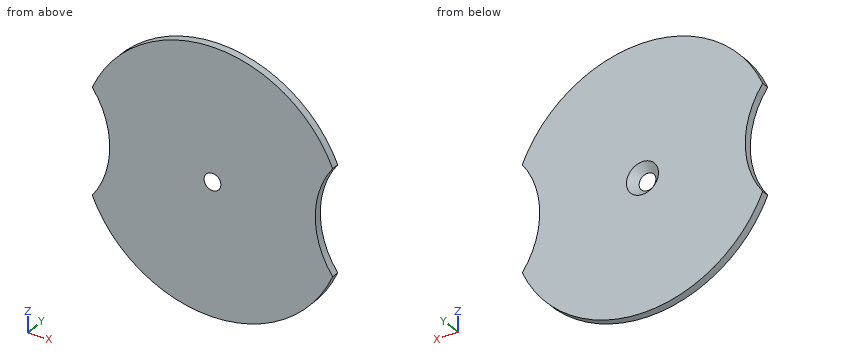
Autodesk Inventor part; units mm, degrees
ref_plane "YZ Plane" through (0, 0, 0) normal (1, 0, 0) x (0, 1, 0)
ref_plane "XZ Plane" through (0, 0, 0) normal (0, 1, 0) x (-1, 0, 0)
ref_plane "XY Plane" through (0, 0, 0) normal (0, 0, 1) x (1, 0, 0)
sketch "スケッチ1" plane through (0, 0, 0) normal (0, 1, 0) x (-1, 0, 0)
  line L0 (0, -24.08) -> (0, 24.08)
  line L1 (-51.0552, 0) -> (51.0552, 0)
  circle A0 centre (0, 0) radius 17.2
  circle A1 centre (0, 0) radius 1.1
  circle A2 centre (24.968, 0) radius 11.5
  circle A3 centre (-24.968, 0) radius 11.5
  line L2 (1.9153, -7.1479) -> (2.64, -9.8524)
  arc A4 (-1.9153, -7.1479) -> (1.9153, -7.1479) centre (0, 0) ccw
  line L3 (-1.9153, -7.1479) -> (-2.64, -9.8524)
  line L4 (0, -11) -> (0.5714, -10.184)
  line L5 (0, -11) -> (-0.5714, -10.184)
  arc A5 (-2.64, -9.8524) -> (-0.5714, -10.184) centre (0, 0) ccw
  arc A6 (0.5714, -10.184) -> (2.64, -9.8524) centre (0, 0) ccw
  point P0 (-15.76, 6.8893)
  point P1 (-15.76, -6.8893)
  point P2 (15.76, -6.8893)
  point P3 (15.76, 6.8893)
  dimension "d0" = 34.4
  dimension "d1" = 2.2
  dimension "d2" = 24.968
  dimension "d3" = 23
  dimension "d8" = 30
  dimension "d9" = 7.4
  dimension "d11" = 10.2
  dimension "d12" = 11
  dimension "d13" = 70
extrude "押し出し1" add sketch "スケッチ1" along normal blind 1 contours A0 A3 L1 A1 L0 A4 L3 A5 L5 | L0 L4 A6 L2 A4 A1 L1 A2 A0 | L5 A5 L3 A4 L0 | L0 A4 L2 A6 L4 | A3 A0 L0 A1 L1 | L1 A1 L0 A0 A2
chamfer "面取り1" distance 1 angle 45 1 edges at (1.1, 1, 0)
properties part number "GearCenterCover"
Here's how the part is built. I have some questions about the finished solid (model axes, mm). Coordinates: 2 decimals unless noted, no trailing zeros. Order: outer loops, then holes, each group sorted by start corner. A loop starts at its lowest first (then second) coordinate and runs counter-clockwise, first axis right, second up.
Item 1: If we section it at D-D, the plane x = -10.5: List the corners of the cut face in (y, z) for me.
Response values:
outline: (0, -13.62) - (1, -13.62) - (1, 13.62) - (0, 13.62) - close
Item 2: If we section it at B-B, the plane y = 0.7: List the corners of the cut face in (x, z) for me, then the cut area to 3 significant figures.
Response values:
outline: (-15.76, -6.89) arc R17.2 ccw to (15.76, -6.89) arc R11.5 cw to (15.76, 6.89) arc R17.2 ccw to (-15.76, 6.89) arc R11.5 cw to start; hole circle Ø3.6 at (0, 0)
area: 850 mm2
Item 3: I'm going to push a flat-ended pin straight in: pin 1 Ø2.5 at (x, z) = (0, 0) entering from +Y. Where does the tip first touch, or does it pass through?
Response values:
pin 1: stops at y = 0.15
Item 4: I need wall thicknesses on probe 1 along X at (y, z) = (0.05, 0); probe 2 along X at (y, z) = (0.4, 8); probe 3 along X at (y, z) = (0.3, 7). Which ranges of each line are inside material? Lowest first, please.
Response values:
probe 1: x = -13.47 to -1.15, 1.15 to 13.47
probe 2: x = -15.23 to 15.23
probe 3: x = -15.71 to 15.71
Item 5: If we section it at C-C, the plane z = -6.5: List the corners of the cut face in (x, y) for me.
Response values:
outline: (-15.48, 0) - (15.48, 0) - (15.48, 1) - (-15.48, 1) - close
